For this review, take the finished solid that the model builds, in its own axes (mm). Give positions to 0.01 mm unless a question says otherwise; leave off trailing zeros. Order: outer loops, then holes, each group sorted by start corner. A loop starts at its lowest first (then second) coordinate and runs counter-clockwise, first axis right, second up.
from build123d import *

# Parameters (mm, degrees)
SKETCH_1_R               = 35
EXTRUDE_1_DEPTH          = 2
CUT_EXTRUDE_1_DEPTH      = 50.537864306
CUT_EXTRUDE_1_DEPTH_BACK = 50.537864306
SKETCH_2_R               = 1.9


with BuildPart() as part:
    # ｽｹｯﾁ1 → ﾎﾞｽ - 押し出し1 (new body)
    with BuildSketch(Plane.XY):
        Circle(SKETCH_1_R)
    extrude(amount=EXTRUDE_1_DEPTH)

    # ｽｹｯﾁ2 → ｶｯﾄ - 押し出し1 (cut, two sides: drawn at the far end of the back side and taken through both)
    with BuildSketch(Plane.XY.offset(-CUT_EXTRUDE_1_DEPTH_BACK)):
        with Locations((0, 30)):
            Circle(SKETCH_2_R)
        with Locations((25.980762114, -15)):
            Circle(SKETCH_2_R)
        with Locations((-25.980762114, -15)):
            Circle(SKETCH_2_R)
        Circle(SKETCH_2_R)
    extrude(amount=CUT_EXTRUDE_1_DEPTH + CUT_EXTRUDE_1_DEPTH_BACK, mode=Mode.SUBTRACT)


solid = part.part
1) To check wall thickness, follow line 1 (Y direction, x = 0, z = 0.9); line 2 (X direction, y = -15, z = 0.45); line 3 (X direction, y = 4, z = 0.9). State the ranges of each line that lie inside material, in increasing order.
Answer sheet:
line 1: y = -35 to -1.9, 1.9 to 28.1, 31.9 to 35
line 2: x = -31.62 to -27.88, -24.08 to 24.08, 27.88 to 31.62
line 3: x = -34.77 to 34.77
2) We need section B-B on x = 0. Give the boundary of the cut face in (y, z), then the cut area to 3 significant figures.
Answer sheet:
outline: (-35, 0) - (-1.9, 0) - (-1.9, 2) - (-35, 2) - close; (1.9, 0) - (28.1, 0) - (28.1, 2) - (1.9, 2) - close; (31.9, 0) - (35, 0) - (35, 2) - (31.9, 2) - close
area: 125 mm2
3) We need section C-C on z = 0.5. Give the boundary of the cut face in (x, y).
Answer sheet:
outline: circle Ø70 at (0, 0); hole circle Ø3.8 at (-25.98, -15); hole circle Ø3.8 at (0, 0); hole circle Ø3.8 at (0, 30); hole circle Ø3.8 at (25.98, -15)
4) Draft analysis for pull direction Y (two halves, no side actions). For faces 1 (the face through (0, -7, 0)), 2 (the face through (-28, -21, 1)), 3 (the face through (-0.247, 31.884, 0.986)), state which applies: +Y half, -Y half, draft (parallel to the pull), parting line (faces both ways), or undercut.
Answer sheet:
face 1: draft
face 2: parting line
face 3: undercut
5) We need section A-A on y = 0. Give the boundary of the cut face in (x, z).
Answer sheet:
outline: (-35, 0) - (-1.9, 0) - (-1.9, 2) - (-35, 2) - close; (1.9, 0) - (35, 0) - (35, 2) - (1.9, 2) - close
6) Clearance check with flat-ended pins moving along their axes: pin 1 (1 mm diameter, centred on x = 18, z = 1, fed in from -Y); pin 2 (3.5 mm diameter, centred on x = -25.98, y = -15, fed in from -Z). State where each tip first meets the part, or that it passes through.
Answer sheet:
pin 1: stops at y = -30.31
pin 2: passes through
7) We need section D-D on y = -15. Give the boundary of the cut face in (x, z).
Answer sheet:
outline: (-31.62, 0) - (-27.88, 0) - (-27.88, 2) - (-31.62, 2) - close; (-24.08, 0) - (24.08, 0) - (24.08, 2) - (-24.08, 2) - close; (27.88, 0) - (31.62, 0) - (31.62, 2) - (27.88, 2) - close
